Answer from the drawing. Dimensions are ordinates in mm from the lowest x, y and z of the part. A direction names the side the tool comes from. Give positions to 0.01 mm unless a question says otherwise; leave off trailing zeros. Order: outer loops, then holes, each group sorted by start corner. A loop starts at its lowest first (then second) coordinate and runs counter-clockwise, first axis right, second up. Notation, with made-up numbers: (1, 60.25) - (8, 60.25) arc R15 ccw to (8, 84.25) - close; hole circle Ø9 at (77, 60). An arc over 180 degrees is marked (long way). Write each question's results on one line, items separated by ' | '.
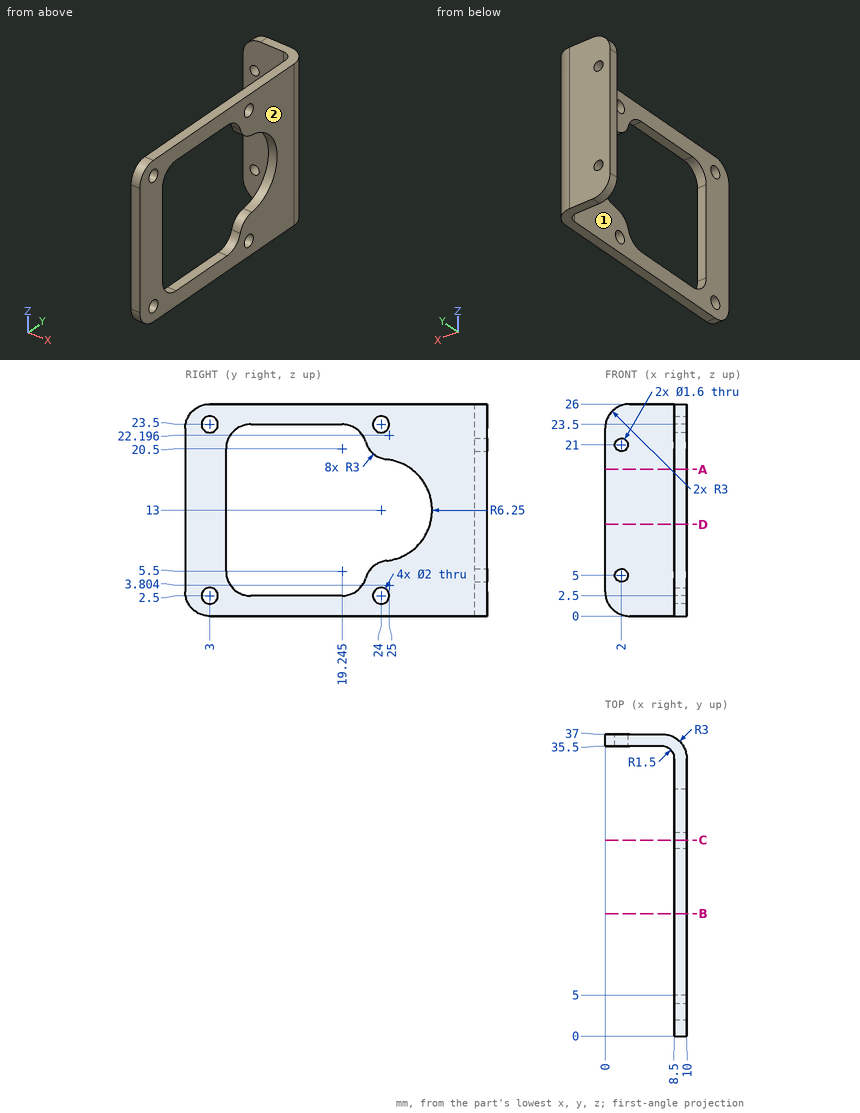
(1) Section B-B (y = 15) is taken. Give the vertices of the cut face in (x, z).
Conclusion:
outline: (8.5, 0) - (10, 0) - (10, 2.5) - (8.5, 2.5) - close; (8.5, 23.5) - (10, 23.5) - (10, 26) - (8.5, 26) - close
(2) For the marked faces 1 and 2, determine the directions among +Z, -Z, +X, -X, +Y, -Y from which every point of the face is accessible in a straight line to the end or side of a thin tool.
Conclusion:
face 1: +Z, -Z, -X, -Y | face 2: +Z, -Z, +X, +Y, -Y
(3) Each of these flat-tipped pins is pushed along its axis until it touches: pin 1 (2.5 mm diameter, centred on y = 3, z = 23.5, fed in from -X); pin 2 (4 mm diameter, centred on y = 33, z = 20, fed in from -X); pin 3 (1.6 mm diameter, centred on x = 9.5, y = 12, fed in from -Z); pin 4 (2 mm diameter, centred on x = 4, z = 14, fed in from -Y). Where does it stop, or does it pass through?
Conclusion:
pin 1: x = 8.5 | pin 2: x = 8.12 | pin 3: z = 0 | pin 4: y = 35.5
(4) Consider probe 1 along Z at (x, y) = (2, 35.95); probe 2 along Y at (x, z) = (6.5, 5); probe 3 along X at (y, z) = (3.5, 4.25). Determine where each line is inside the solid, lowest interval first. Write a range as [from, to].
Conclusion:
probe 1: [0.17, 4.2], [5.8, 20.2], [21.8, 25.83] | probe 2: [35.5, 37] | probe 3: [8.5, 10]
(5) Section D-D (z = 11.25) is taken. Give the vertices of the cut face in (x, y), plus the area to 3 significant figures.
Conclusion:
outline: (0, 35.5) - (7, 35.5) arc R1.5 cw to (8.5, 34) - (8.5, 30) - (10, 30) - (10, 34) arc R3 ccw to (7, 37) - (0, 37) - close; (8.5, 0) - (10, 0) - (10, 5) - (8.5, 5) - close | area: 29.3 mm^2
(6) Section C-C (y = 24) is taken. Give the vertices of the cut face in (x, z), plus the area to 3 significant figures.
Conclusion:
outline: (8.5, 0) - (10, 0) - (10, 1.5) - (8.5, 1.5) - close; (8.5, 3.5) - (10, 3.5) - (10, 6.63) - (8.5, 6.63) - close; (8.5, 19.37) - (10, 19.37) - (10, 22.5) - (8.5, 22.5) - close; (8.5, 24.5) - (10, 24.5) - (10, 26) - (8.5, 26) - close | area: 13.9 mm^2
(7) Section A-A (z = 18) is taken. Give the vertices of the cut face in (x, y).
Conclusion:
outline: (0, 35.5) - (7, 35.5) arc R1.5 cw to (8.5, 34) - (8.5, 27.75) - (10, 27.75) - (10, 34) arc R3 ccw to (7, 37) - (0, 37) - close; (8.5, 0) - (10, 0) - (10, 5) - (8.5, 5) - close
